Autodesk Inventor part; units mm, degrees
ref_plane "YZ Plane" through (0, 0, 0) normal (1, 0, 0) x (0, 1, 0)
ref_plane "XZ Plane" through (0, 0, 0) normal (0, 1, 0) x (-1, 0, 0)
ref_plane "XY Plane" through (0, 0, 0) normal (0, 0, 1) x (1, 0, 0)
sketch "스케치13" plane through (0, 0, 0) normal (0, 0, 1) x (1, 0, 0)
  circle A0 centre (0, 0) radius 35
  dimension "d74" = 70
extrude "돌출11" add sketch "스케치13" along normal blind 7
sketch "스케치19" plane through (0, 0, 7) normal (0, 0, 1) x (1, 0, 0)
  circle A0 centre (0, 0) radius 20
  dimension "d92" = 40
extrude "돌출17" add sketch "스케치19" along normal blind 3
sketch "스케치20" plane through (0, 0, 10) normal (0, 0, 1) x (1, 0, 0)
  circle A0 centre (0, 0) radius 16
  dimension "d95" = 32
extrude "돌출18" cut sketch "스케치20" against normal blind 5
sketch "스케치16" plane through (0, 0, 0) normal (0, 0, -1) x (-1, 0, 0)
  circle A0 centre (0, 0) radius 23.5
  dimension "d83" = 47
extrude "돌출15" add sketch "스케치16" along normal blind 3
sketch "스케치23" plane through (0, 0, -3) normal (0, 0, -1) x (-1, 0, 0)
  circle A0 centre (0, 0) radius 18.5
  dimension "d117" = 37
extrude "돌출20" cut sketch "스케치23" against normal blind 3
sketch "스케치18" plane through (0, 0, -3) normal (0, 0, -1) x (-1, 0, 0)
  circle A0 centre (0, 0) radius 10.5
  dimension "d89" = 21
extrude "돌출16" cut sketch "스케치18" against normal up to next
sketch "스케치21" plane through (0, 0, 7) normal (0, 0, 1) x (1, 0, 0)
  circle A0 centre (0, 28) radius 4
  line L0 (-4, 28) -> (4, 28)
  line L1 (4, 28) -> (4, 38)
  line L2 (4, 38) -> (-4, 38)
  line L3 (-4, 38) -> (-4, 28)
  point P0 (0, 0)
  dimension "d99" = 8
  dimension "d100" = 28
extrude "돌출19" cut sketch "스케치21" against normal blind 4.4
sketch "스케치22" plane through (0, 0, 2.6) normal (0, 0, 1) x (1, 0, 0)
  arc A0 (-4, 28) -> (4, 28) centre (0, 28) ccw
  circle A1 centre (0, 28) radius 4
  point P0 (0, 0)
hole "구멍2" at (0, 28, 2.6) direction (0, 0, -1) diameter 4.5 end through all
fillet "모깎기7" radius 3 4 edges at (-23.2916, -26.1247, 7) (26.1247, 23.2916, 7) (-20, 0, 10) (18.5, 0, 0)
chamfer "모따기6" distance 1 angle 45 1 edges at (23.5, 0, -3)
properties part number "도면3-2번"
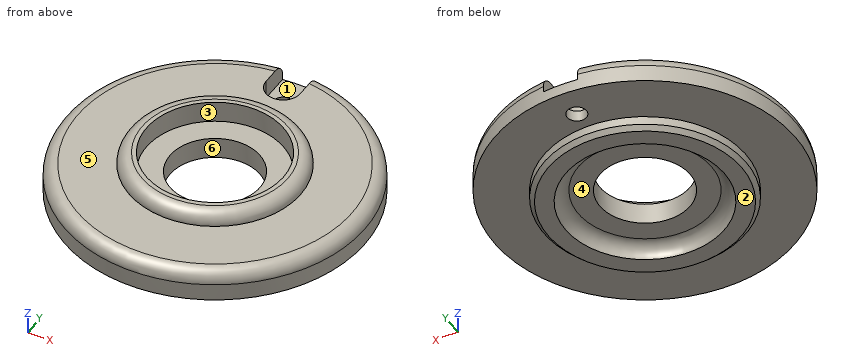
Work out the finished part from the listing and answer in its coordinate system (mm). Face numbers are marked on the shaded views. A direction names the side the tool comes from. Coordinates: 2 decimals unless noted, no trailing zeros. Use a Markdown table: item, result.
Item 1: Consider probe 1 along Y at (x, z) = (0, 1.65); probe 2 along Z at (x, y) = (-11.5, 4); probe 3 along X at (y, z) = (28, 1.5). Determine where each line is inside the solid, lowest interval first. Write a range as from..to.
Evaluation:
| item | result |
|---|---|
| probe 1 | y = -35..-10.5, 10.5..25.75, 30.25..35 |
| probe 2 | z = 0..5 |
| probe 3 | x = -21..-2.25, 2.25..21 |
Item 2: Given pin 1 Ø24 at (x, y) = (0, 0) entering from -Z; pin 2 Ø1 at (x, y) = (-24, -12) entering from +Z; pin 3 Ø1.5 at (y, z) = (12, 4.5) entering from -X; pin 4 Ø6 at (x, z) = (1, 4.5) entering from -Y, each flat-ended and moving along its own axis, determine where each tip first touches the part or whether it passes through.
Evaluation:
| item | result |
|---|---|
| pin 1 | stops at z = 0 |
| pin 2 | stops at z = 7 |
| pin 3 | stops at x = -33.12 |
| pin 4 | stops at y = -35 |
Item 3: The mould has two halves that part along Y. Classify the marked faces 5 and 6: +Y half, -Y half, draft (parallel to the pull), parting line (faces both ways), or undercut.
Evaluation:
| item | result |
|---|---|
| face 5 | draft |
| face 6 | undercut |
Item 4: Find section A-A, the plane x = 0. State how many separate pieces and enclosed holes the cut face has, and give its area (3 significant figures).
Evaluation:
| item | result |
|---|---|
| separate pieces | 3 |
| enclosed holes | 0 |
| area | 312 mm2 |
Item 5: For the marked faces 1, 2, 3 and 4, determine the directions among +Z, -Z, +X, -X, +Y, -Y from which every point of the face is accessible in a straight line to the end or side of a thin tool.
Evaluation:
| item | result |
|---|---|
| face 1 | +Z, +Y |
| face 2 | -Z, +X, -X, +Y, -Y |
| face 3 | +Z |
| face 4 | -Z |
